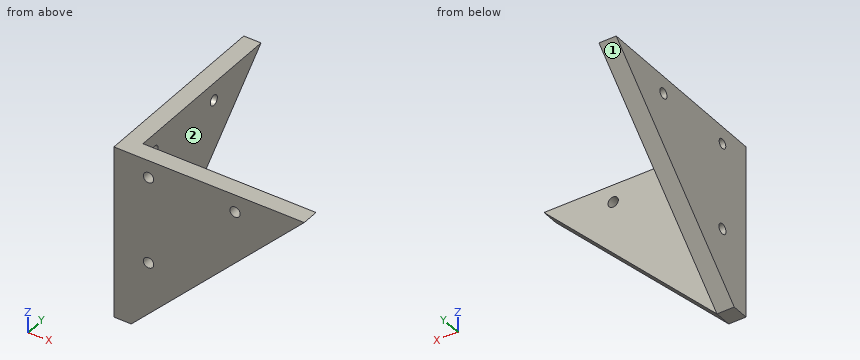
```python
from build123d import *

# Parameters (mm, degrees)
EXTRUDE_1_DEPTH     = 5
EXTRUDE_2_DEPTH     = 5
SKETCH_4_W          = 5
SKETCH_4_H          = 5
EXTRUDE_4_DEPTH     = 50
EXTRUDE_13_DEPTH    = 5
SKETCH_8_R          = 1.5
SKETCH_8_R_2        = 1.4
CUT_EXTRUDE_1_DEPTH = 87.602540378
SKETCH_9_R          = 1.5
CUT_EXTRUDE_2_DEPTH = 87.602540378
SKETCH_10_R         = 1.5
CUT_EXTRUDE_3_DEPTH = 87.602540378
CUT_EXTRUDE_4_DEPTH = 5


with BuildPart() as part:
    # Sketch 1 → Extrude 1 (new body)
    with BuildSketch(Plane.XY):
        Polygon((0, 50), (50, 0), (50, -5), (-5, -5), (-5, 50), align=None)
    extrude(amount=EXTRUDE_1_DEPTH)



with BuildPart() as body_2:
    # Sketch 2 → Extrude 2 (new body)
    with BuildSketch(Plane(origin=(0, 0, 0), x_dir=(0, 0, -1), z_dir=(1, 0, 0))):
        Polygon((0, 0), (50, 0), (0, 50), align=None)
    extrude(amount=-EXTRUDE_2_DEPTH)

    # Sketch 4 → Extrude 4 (add)
    with BuildSketch(Plane.XY):
        with Locations((-2.5, -2.5)):
            Rectangle(SKETCH_4_W, SKETCH_4_H)
    extrude(amount=-EXTRUDE_4_DEPTH)


with BuildPart() as part_1:
    add(part.part)

    add(body_2.part)  # Extrude 13 merges body 2
    # Sketch 7 → Extrude 13 (add)
    with BuildSketch(Plane.XZ.offset(5)):
        Polygon((50, 0), (0, 0), (0, -50), align=None)
    extrude(amount=-EXTRUDE_13_DEPTH)

    # Sketch 8 → Cut-Extrude 1 (cut, through all)
    with BuildSketch(Plane(origin=(0, 0, 0), x_dir=(0, 0, -1), z_dir=(1, 0, 0))):
        with Locations((5, 30)):
            Circle(SKETCH_8_R)
        with Locations((5, 5)):
            Circle(SKETCH_8_R_2)
        with Locations((30, 5)):
            Circle(SKETCH_8_R)
    extrude(amount=-CUT_EXTRUDE_1_DEPTH, mode=Mode.SUBTRACT)

    # Sketch 9 → Cut-Extrude 2 (cut, through all)
    with BuildSketch(Plane(origin=(0, 0, 0), x_dir=(-1, 0, 0), z_dir=(0, 0, -1))):
        with Locations((-5, 30)):
            Circle(SKETCH_9_R)
        with Locations((-5, 5)):
            Circle(SKETCH_9_R)
        with Locations((-30, 5)):
            Circle(SKETCH_9_R)
    extrude(amount=-CUT_EXTRUDE_2_DEPTH, mode=Mode.SUBTRACT)

    # Sketch 10 → Cut-Extrude 3 (cut, through all)
    with BuildSketch(Plane(origin=(0, 0, 0), x_dir=(1, 0, 0), z_dir=(0, 1, 0))):
        with Locations(Location((5, 30, 0), (0, 0, 270))):
            Circle(SKETCH_10_R)
        with Locations(Location((5, 5, 0), (0, 0, 270))):
            Circle(SKETCH_10_R)
        with Locations(Location((30, 5, 0), (0, 0, 270))):
            Circle(SKETCH_10_R)
    extrude(amount=-CUT_EXTRUDE_3_DEPTH, mode=Mode.SUBTRACT)

    # Sketch 11 → Cut-Extrude 4 (cut)
    with BuildSketch(Plane.XY.offset(5)):
        Polygon((-5, 50), (-5, -5), (50, -5), (50, 0), (0, 50), align=None)
    extrude(amount=-CUT_EXTRUDE_4_DEPTH, mode=Mode.SUBTRACT)


solid = part_1.part
```
The listing builds one solid part. Answer for the finished solid, in the listing's coordinates (mm). Face numbers are marked on the shaded views. A direction names the side the tool comes from. Coordinates: 2 decimals unless noted, no trailing zeros. Write each loop counter-clockwise with the first axis right and the second up, starting at its lowest first coordinate (ties: lowest second). Pieces come first, ordered by that corner, then holes. Notation, with made-up numbers: (65.25, 71.5) - (77.25, 71.5) arc R15 cw to (77.25, 94.5) - close; hole circle Ø2 at (10, 15). An arc over 180 degrees is marked (long way). Return JSON: item names as keys, results as strings. Group by question number.
Q1. The part is cut by section C-C on x = 5. Write down the section's boundary in (y, z).
Q2. Find the intervals of material crossed by line 1 along Y through (x, z) = (-1, -5); line 2 along Y through (x, z) = (7, -17), in increasing order. Write a range as [from, to].
Q3. The part is cut by section A-A on z = -30. Write down the section's boundary in (x, y), and give its area (3 significant figures).
Q4. The part is cut by section D-D on z = -5. Write down the section's boundary in (x, y).
Q5. Which of the six approach directions +Z, -Z, +X, -X, +Y, -Y give full straight-line access (tool end or side, diameter ignored) to the marked faces 1 and 2?
Q6. Flat-ended cylindrical pins translate along their axes: pin 1 Ø1.7 at (y, z) = (5, -5) entering from +X; pin 2 Ø3.5 at (x, z) = (30, -5) entering from +Y; pin 3 Ø25 at (y, z) = (19, -32.5) entering from +X. Find the tip coordinate at first contact, or state that the pin passes through.
Q7. The part is cut by section B-B on y = 5. Write down the section's boundary in (x, z).
Evaluation:
{
 "1": {"outline": "(-5, -45) - (0, -45) - (0, -31.5) - (-5, -31.5) - close; (-5, -28.5) - (0, -28.5) - (0, -6.5) - (-5, -6.5) - close; (-5, -3.5) - (0, -3.5) - (0, 0) - (-5, 0) - close"},
 "2": {"line 1": "y = [-5, 3.6], [6.4, 28.5], [31.5, 45]", "line 2": "y = [-5, 0]"},
 "3": {"outline": "(-5, -5) - (3.5, -5) - (3.5, 0) - (0, 0) - (0, 3.5) - (-5, 3.5) - close; (-5, 6.5) - (0, 6.5) - (0, 20) - (-5, 20) - close; (6.5, -5) - (20, -5) - (20, 0) - (6.5, 0) - close", "area": "195 mm2"},
 "4": {"outline": "(-5, -5) - (3.5, -5) - (3.5, 0) - (0, 0) - (0, 3.6) - (-5, 3.6) - close; (-5, 6.4) - (0, 6.4) - (0, 28.5) - (-5, 28.5) - close; (-5, 31.5) - (0, 31.5) - (0, 45) - (-5, 45) - close; (6.5, -5) - (28.5, -5) - (28.5, 0) - (6.5, 0) - close; (31.5, -5) - (45, -5) - (45, 0) - (31.5, 0) - close"},
 "5": {"face 1": "-Z, +X, -X, +Y", "face 2": "+Z, -Z, +X, +Y"},
 "6": {"pin 1": "passes through", "pin 2": "stops at y = 0", "pin 3": "stops at x = 0"},
 "7": {"outline": "(-5, -45) - (0, -45) - (0, -31.5) - (-5, -31.5) - close; (-5, -28.5) - (0, -28.5) - (0, -6.4) - (-5, -6.4) - close; (-5, -3.6) - (0, -3.6) - (0, 0) - (-5, 0) - close"}
}
